from build123d import *

# Parameters (mm, degrees)
F0_R     = 5
F1_DEPTH = 4
F2_R     = 2.75
F3_DEPTH = 2.5
F4_SIZE  = 0.5


with BuildPart() as f1:
    # F0 (on Top) → F1 (new body)
    with BuildSketch(Plane.XY):
        Circle(F0_R)
    extrude(amount=F1_DEPTH)

    # F2 (on face) → F3 (cut)
    with BuildSketch(Plane.XY.offset(4)):
        Circle(F2_R)
    extrude(amount=-F3_DEPTH, mode=Mode.SUBTRACT)

    # F4
    f4_edges = [f1.edges().sort_by_distance(p)[0] for p in [
        (-2.75, 0, 4),
        (-5, 0, 0),
    ]]
    chamfer(f4_edges, length=F4_SIZE)


solid = f1.part
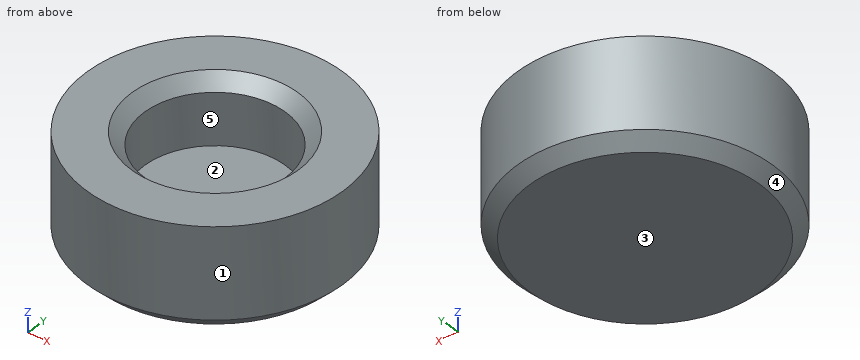
Geometry: final body of the model. Coordinates: model frame, mm. Face numbers are marked on the shaded views. A direction names the side the tool comes from. Round coordinates to 2 decimals unless told otherwise and drop trailing zeros. Order: outer loops, then holes, each group sorted by start corner. A loop starts at its lowest first (then second) coordinate and runs counter-clockwise, first axis right, second up.
Q1. Pin query (flat end, axial travel): pin 1 (3 mm diameter, centred on x = -0.5, y = 0, fed in from +Z); pin 2 (5 mm diameter, centred on x = 3, y = -3, fed in from -Z); pin 3 (1 mm diameter, centred on x = -1.5, z = 1.5, fed in from -Y). Return the tip coordinate at first contact, or that it passes through.
Result sheet:
pin 1: stops at z = 1.5
pin 2: stops at z = 0
pin 3: stops at y = -4.9
Q2. Section C-C, the plane z = 1.65. Output: boundary loops of the cut face in (x, y).
Result sheet:
outline: circle Ø10 at (0, 0); hole circle Ø5.5 at (0, 0)
Q3. Access query for the marked faces 1 and 2. Directions: +Z, -Z, +X, -X, +Y, -Y. A direction counts if a zero-diameter tool reaches every point of the face in a straight line with its end or side. Return the directions, or none.
Result sheet:
face 1: +Z, -Z
face 2: +Z
Q4. Mould query, pull axis Y, two halves, no side actions, for the marked faces 3, 4 and 5. Classes: released by +Y, released by -Y, zero draft, split by the parting line, or undercut.
Result sheet:
face 3: zero draft
face 4: split by the parting line
face 5: undercut
Q5. Material intervals for probe 1 along Y at (x, z) = (0, 3); probe 2 along Z at (x, y) = (-1.75, -0.75); probe 3 along X at (y, z) = (-2.25, 1.6), sorted ascending.
Result sheet:
probe 1: y = -5 to -2.75, 2.75 to 5
probe 2: z = 0 to 1.5
probe 3: x = -4.47 to -1.58, 1.58 to 4.47
Q6. Section A-A, the plane y = 0. Output: boundary loops of the cut face in (x, z), and give its area (4 significant figures).
Result sheet:
outline: (-5, 0.5) - (-4.5, 0) - (4.5, 0) - (5, 0.5) - (5, 4) - (3.25, 4) - (2.75, 3.5) - (2.75, 1.5) - (-2.75, 1.5) - (-2.75, 3.5) - (-3.25, 4) - (-5, 4) - close
area: 25.75 mm2
Q7. Section D-D, the plane z = 0.3. Output: boundary loops of the cut face in (x, y).
Result sheet:
outline: circle Ø9.6 at (0, 0)
